Can you work these out from the model? Positions are in its coordinate system, mm. Give positions to 0.01 mm unless a question says otherwise; leave off trailing zeros. Order: outer loops, then holes, each group sorted by start corner. A loop starts at its lowest first (then second) coordinate and runs counter-clockwise, first axis right, second up.
Item 1: I want a section at A-A, the plane x = -265.5. Write out the boundary of the cut face in (y, z), then the cut area to 3 significant figures.
Item 2: If I drill on line 1 along Y through (x, z) = (-264, 1.95); line 2 along X through (y, z) = (96.5, 0.3), over which ranges is the centre line in solid material (lowest first)?
Item 3: I'm going to push flat-ended pins straight in: pin 1 Ø3 at (x, y) = (-333, 117) entering from -Z; pin 2 Ø1.5 at (x, z) = (-172.5, 1) entering from -Y; pin 3 Ø1.5 at (y, z) = (71.5, 1.5) entering from +X; pin 4 Ø0.9 at (x, z) = (-380, 1.5) entering from +Y. Where does each tip first touch, or does it pass through?
Item 4: I want a section at B-B, the plane y = 92. Write out the boundary of the cut face in (x, z).
```python
from build123d import *

# Parameters (mm, degrees)
BOSS_EXTRUDE1_DEPTH = 3
SKETCH3_W           = 3
SKETCH3_H           = 12
BOSS_EXTRUDE2_DEPTH = 3


with BuildPart() as part:
    # Sketch2 → Boss-Extrude1 (new body)
    with BuildSketch(Plane(origin=(-276.446036152, 132.735684364, 0), x_dir=(1, 0, 0), z_dir=(0, 0, 1))):
        Polygon((-78, 3), (-78, 0), (-90, 0), (-90, 3), (-102.5, 3), (-102.5, -62.99938194), (-90, -62.99938194), (-90, -59.99938194), (-78, -59.99938194), (-78, -62.99938194), (-66, -62.99938194), (-66, -59.99938194), (-54, -59.99938194), (-54, -62.99938194), (-42, -62.99938194), (-42, -59.99938194), (-30, -59.99938194), (-30, -62.99938194), (-18, -62.99938194), (-18, -59.99938194), (-6, -59.99938194), (-6, -62.99938194), (6, -62.99938194), (6, -59.99938194), (18, -59.99938194), (18, -62.99938194), (30, -62.99938194), (30, -59.99938194), (42, -59.99938194), (42, -62.99938194), (54, -62.99938194), (54, -59.99938194), (66, -59.99938194), (66, -62.99938194), (78, -62.99938194), (78, -59.99938194), (90, -59.99938194), (90, -62.99938194), (102.5, -62.99938194), (102.5, 3), (90, 3), (90, 0), (78, 0), (78, 3), (66, 3), (66, 0), (54, 0), (54, 3), (42, 3), (42, 0), (30, 0), (30, 3), (18, 3), (18, 0), (6, 0), (6, 3), (-6, 3), (-6, 0), (-18, 0), (-18, 3), (-30, 3), (-30, 0), (-42, 0), (-42, 3), (-54, 3), (-54, 0), (-66, 0), (-66, 3), align=None)
    extrude(amount=BOSS_EXTRUDE1_DEPTH)

    # Sketch3 → Boss-Extrude2 (add)
    with BuildSketch(Plane(origin=(-276.446036152, 132.735684364, 3), x_dir=(1, 0, 0), z_dir=(0, 0, 1))):
        with Locations((-104, -6)):
            Rectangle(SKETCH3_W, SKETCH3_H)
        with Locations((104, -6)):
            Rectangle(SKETCH3_W, SKETCH3_H)
        with Locations((104, -30)):
            Rectangle(SKETCH3_W, SKETCH3_H)
        with Locations((104, -54)):
            Rectangle(SKETCH3_W, SKETCH3_H)
        with Locations((-104, -30)):
            Rectangle(SKETCH3_W, SKETCH3_H)
        with Locations((-104, -54)):
            Rectangle(SKETCH3_W, SKETCH3_H)
    extrude(amount=-BOSS_EXTRUDE2_DEPTH)


solid = part.part
```
Results list:
1. outline: (72.74, 0) - (132.74, 0) - (132.74, 3) - (72.74, 3) - close
1. area: 180 mm2
2. line 1: y = 72.74 to 132.74
2. line 2: x = -378.95 to -173.95
3. pin 1: stops at z = 0
3. pin 2: stops at y = 72.74
3. pin 3: stops at x = -173.95
3. pin 4: stops at y = 132.74
4. outline: (-378.95, 0) - (-173.95, 0) - (-173.95, 3) - (-378.95, 3) - close
